Read the model definition and answer for the solid it produces. Units are mm, in the model's axes. Face numbers are marked on the shaded views. A direction names the side the tool comes from. Coordinates: 2 decimals unless noted, no trailing zeros. Order: outer loops, then holes, each group sorted by start corner. A loop starts at its lowest first (then second) coordinate and runs counter-clockwise, first axis right, second up. Notation, with made-up numbers: M 29.5,68 L 66.5,68 A21 ccw 66.5,77 Z; hole C 75.5,4 d2. An arc over 180 degrees is marked long. One line per question, with ' | ' between items. Start each with the question number.
1) Find section D-D, the plane x = -26. Write down the section's boundary in (y, z).
2) Consider probe 1 along Y at (x, z) = (30.5, 35); probe 2 along Z at (x, y) = (34, 2.75); probe 3 along Z at (x, y) = (3.5, 2). Determine where each line is inside the solid, lowest interval first.
3) Find section B-B, the plane y = 2.5. Write down the section's boundary in (x, z) (1 decimal).
4) A tool of negligible diameter and unlimited length cuts with its end or side. For the marked faces 1 and 2, from which of +Z, -Z, +X, -X, +Y, -Y can it reach the whole face along a straight path? Write none if from no direction.
5) Find section C-C, the plane z = -22.86. Write down the section's boundary in (x, y) (3 decimals).
6) Given P1, Ø3.5, axis at x = -39.59, z = -22.86, coming from the +Y side; P2, Ø4.5, axis at x = 45.72, z = 0, coming from the -Y side; P3, Ø1, axis at x = -39, z = -23, coming from the +Y side (3 decimals); P4, Ø3, axis at y = 4.5, z = 15.5, coming from the +X side, each flat-ended and moving along its own axis, determine where each tip first touches the part or whether it passes through.
from build123d import *

# Parameters (mm, degrees)
F0_R     = 50.8
F1_DEPTH = 6.35
F2_R     = 50.8
F2_R_2   = 37.2745
F3_DEPTH = 2.54
F4_R     = 2.54
F4_R_2   = 1.35255
F5_DEPTH = 6.351
F7_DEPTH = 6.351
F8_R     = 1.5875
F9_DEPTH = 3.175


with BuildPart() as f1:
    # F0 (on Front) → F1 (new body)
    with BuildSketch(Plane.XZ):
        Circle(F0_R)
    extrude(amount=-F1_DEPTH)

    # F2 (on face) → F3 (cut)
    with BuildSketch(Plane(origin=(0, 6.35, 0), x_dir=(-1, 0, 0), z_dir=(0, 1, 0))):
        Circle(F2_R)
        Circle(F2_R_2, mode=Mode.SUBTRACT)
    extrude(amount=-F3_DEPTH, mode=Mode.SUBTRACT)

    # F4 (on face) → F5 (cut, through all)
    with BuildSketch(Plane.XZ):
        Circle(F4_R)
        with Locations((-45.72, 0)):
            Circle(F4_R_2)
        with Locations((45.72, 0)):
            Circle(F4_R_2)
    extrude(amount=-F5_DEPTH, mode=Mode.SUBTRACT)

    # F6 (on face) → F7 (cut, through all)
    with BuildSketch(Plane.XZ):
        with BuildLine():
            ThreePointArc((9.7364788506, -32.6571428571), (0, -25.4), (-9.7364788506, -32.6571428571))
            Line((-9.7364788506, -32.6571428571), (-14.5142857143, -48.682394253))
            ThreePointArc((-14.5142857143, -48.682394253), (0, -50.8), (14.5142857143, -48.682394253))
            Line((14.5142857143, -48.682394253), (9.7364788506, -32.6571428571))
        make_face()
    extrude(amount=-F7_DEPTH, mode=Mode.SUBTRACT)

    # F8 (on face) → F9 (cut)
    with BuildSketch(Plane(origin=(0, 3.81, 0), x_dir=(-1, 0, 0), z_dir=(0, 1, 0))):
        with Locations((0, 45.72)):
            Circle(F8_R)
        with Locations((39.594681461, -22.86)):
            Circle(F8_R)
        with Locations((-39.594681461, -22.86)):
            Circle(F8_R)
    extrude(amount=-F9_DEPTH, mode=Mode.SUBTRACT)


solid = f1.part
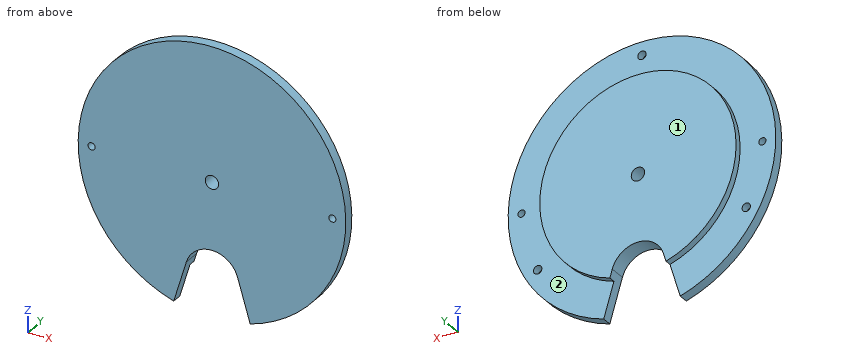
Report:
1) outline: M 0,-43.64 L 3.81,-43.64 L 3.81,-26.71 L 6.35,-26.71 L 6.35,26.71 L 3.81,26.71 L 3.81,43.64 L 0,43.64 Z
2) probe 1: y = 0 to 3.81 | probe 2: z = -37.74 to 37.74 | probe 3: z = -26.02 to 50.68
3) outline: M -14.5,-48.7 L -9.7,-32.7 A10.2 cw 9.7,-32.7 L 14.5,-48.7 A50.8 ccw long Z; hole C -45.7,0 d2.7; hole C -39.6,-22.9 d3.2; hole C 0,0 d5.1; hole C 0,45.7 d3.2; hole C 39.6,-22.9 d3.2; hole C 45.7,0 d2.7
4) face 1: +Z, -Z, +X, -X, +Y | face 2: +Y
5) outline: M -45.366,0 L 45.366,0 L 45.366,3.81 L 41.182,3.81 L 41.182,0.635 L 38.007,0.635 L 38.007,3.81 L 29.442,3.81 L 29.442,6.35 L -29.442,6.35 L -29.442,3.81 L -38.007,3.81 L -38.007,0.635 L -41.182,0.635 L -41.182,3.81 L -45.366,3.81 Z
6) P1: stops at y = 3.81 | P2: stops at y = 0 | P3: stops at y = 0.635 | P4: stops at x = 48.78
